Input: part model. Units: mm. Frame: model coordinates. A direction names the side the tool comes from. Give positions to 0.01 mm unless a question says otherwise; leave off trailing zeros. Write each loop counter-clockwise with the first axis right and the second up, starting at its lowest first coordinate (ties: lowest second). Pieces come first, ordered by that corner, then holes. Notation, with made-up numbers: (-31.5, 21) - (-23.5, 21) arc R28 ccw to (-23.5, 43) - close; hole circle Ø11 at (-40, 7.5). An arc over 180 degrees is marked (long way). Answer as CSV lines item,"result". Start each with the question number.
from build123d import *

# Parameters (mm, degrees)
BOSS_EXTRU_2_DEPTH      = 100
ENL_V_MAT_EXTRU_1_REACH = 72
ESQUISSE2_W             = 100
ESQUISSE2_H             = 60


with BuildPart() as part:
    # Esquisse1 → Boss.-Extru.2 (new body)
    with BuildSketch(Plane.XY):
        Polygon((0, 0), (150, 0), (90, 70), (30, 70), align=None)
        Polygon((36.59396158, 60), (15.165390151, 10), (128.257793632, 10), (85.400650775, 60), align=None, mode=Mode.SUBTRACT)
    extrude(amount=-BOSS_EXTRU_2_DEPTH)

    # Esquisse2 → Enlèv. mat.-Extru.1 (cut, up to next)
    with BuildSketch(Plane(origin=(0, 70, 0), x_dir=(1, 0, 0), z_dir=(0, 1, 0)), mode=Mode.PRIVATE) as enl_v_mat_extru_1_sk1:
        with Locations((100, 50)):
            Rectangle(ESQUISSE2_W, ESQUISSE2_H)
    enl_v_mat_extru_1_tool1 = extrude(enl_v_mat_extru_1_sk1.sketch, amount=-ENL_V_MAT_EXTRU_1_REACH, mode=Mode.PRIVATE) & part.part
    add(enl_v_mat_extru_1_tool1.solids().sort_by_distance((100, 70, -50))[0], mode=Mode.SUBTRACT)


solid = part.part
1) Pull-direction query (X, two-part tool) for faces 1 (the flat face through (103, 40, -20)), 2 (the flat face through (107.13, 34.65, -89.86)), 3 (the flat face through (50, 5, -50)); classes: +X half, -X half, draft (parallel to the pull), parting line (faces both ways), or undercut.
2) Cut plane B-B on x = 73.5. Output: boundary loops of the cut face in (y, z), and give its area (3 significant figures).
3) Cut plane A-A on x = 43. Output: boundary loops of the cut face in (y, z).
4) Cut plane C-C on z = -76. Output: boundary loops of the cut face in (x, y), and give its area (3 significant figures).
5) Contact query for flat-ended pins moving along their axis: P1, Ø3, axis at y = 5.5, z = -35, coming from the +X side; P2, Ø12, axis at y = 47.5, z = -40, coming from the +X side; P3, Ø1, axis at y = 57.5, z = -42, coming from the +X side. Output: stop coordinate, or through.
6) Cut plane D-D on y = 17. Output: boundary loops of the cut face in (x, z).
7) Reachability of faces 4 (the flat face through (46, 10, -49)), 5 (the flat face through (69, 9, -100)), 6 (the flat face through (50, 65, -50)) from +Z, -Z, +X, -X, +Y, -Y: full face, straight path, thin tool, end or side. Return the list, or none.
8) Material intervals for line 1 (Z direction, x = 115, y = 33); line 2 (Y direction, x = 48, z = -28.5); line 3 (X direction, y = 25, z = -7.5), sorted ascending. Write a range as from..to.
Numbers:
1,face 1,"draft"
1,face 2,"undercut"
1,face 3,"+X half"
2,outline,"(0, -100) - (10, -100) - (10, -80) - (0, -80) - close; (0, -20) - (10, -20) - (10, 0) - (0, 0) - close; (60, -100) - (70, -100) - (70, -80) - (60, -80) - close; (60, -20) - (70, -20) - (70, 0) - (60, 0) - close"
2,area,"800 mm²"
3,outline,"(0, -100) - (10, -100) - (10, 0) - (0, 0) - close; (60, -100) - (70, -100) - (70, 0) - (60, 0) - close"
4,outline,"(0, 0) - (50, 0) - (50, 10) - (15.17, 10) - (36.59, 60) - (50, 60) - (50, 70) - (30, 70) - close"
4,area,"1,240 mm²"
5,P1,"stops at x = 50"
5,P2,"stops at x = 33.81"
5,P3,"stops at x = 35.74"
6,outline,"(7.29, -100) - (18.17, -100) - (18.17, 0) - (7.29, 0) - close; (122.26, -100) - (135.43, -100) - (135.43, -80) - (122.26, -80) - close; (122.26, -20) - (135.43, -20) - (135.43, 0) - (122.26, 0) - close"
7,face 4,"+Z, -Z"
7,face 5,"-Z, +X, -X, +Y, -Y"
7,face 6,"+X, +Y, -Y"
8,line 1,"z = -100..-80, -20..0"
8,line 2,"y = 0..10, 60..70"
8,line 3,"x = 10.71..21.59, 115.4..128.57"
